Input: part model. Units: mm. Frame: model coordinates. Face numbers are marked on the shaded views. Coordinates: 2 decimals unless noted, no trailing zeros. Loops run counter-clockwise (first coordinate to the right, second up) from the corner with the lowest first, then second, coordinate; pieces in that order, holes last. Notation, with made-up numbers: (13.25, 27.25) -> (35.25, 27.25) arc R18 ccw to (35.25, 55.25) -> close; hole circle Ø3 at (78, 41). An arc over 180 degrees is marked (long way). Answer as a JSON object with one key per item and string values.
Autodesk Inventor part; units mm, degrees
ref_plane "YZ Plane" through (0, 0, 0) normal (1, 0, 0) x (0, 1, 0)
ref_plane "XZ Plane" through (0, 0, 0) normal (0, 1, 0) x (-1, 0, 0)
ref_plane "XY Plane" through (0, 0, 0) normal (0, 0, 1) x (1, 0, 0)
sketch "Эскиз1" plane through (0, 0, 0) normal (0, 1, 0) x (-1, 0, 0)
  circle A0 centre (0, 0) radius 2.5
  circle A1 centre (0, 0) radius 7.5
  line L0 (0, 7.5) -> (7.5, 7.5)
  line L1 (7.5, 7.5) -> (7.5, -7.5)
  line L2 (7.5, -7.5) -> (0, -7.5)
  line L3 (0, -7.5) -> (0, 7.5)
  line L4 (-7.5, 0) -> (-12.5, 0)
  circle A2 centre (-12.5, 0) radius 2.6
  circle A3 centre (-12.5, 0) radius 5
  line L5 (-1.5661, 7.3347) -> (-13.4999, 4.899)
  line L6 (-13.5, -4.899) -> (-1.5, -7.3485)
  dimension "d0" = 5
  dimension "d1" = 15
  dimension "d2" = 5
  dimension "d3" = 5.2
extrude "Выдавливание1" add sketch "Эскиз1" along normal blind 2 contours A0 L3 A1 | A0 L3 A1 | L0 L1 A1 | A1 L1 L2 | A1 A3 L5 | L6 A3 A1 | A3
fillet "Сопряжение1" radius 0.7 8 edges at (0.7874, 0, 7.4586) (-3.75, 0, 7.5) (-7.5, 0, 0) (0.7538, 0, -7.462) (7.5, 0, -6.1237) (17.5, 0, 0.0001) (7.533, 0, 6.1168) (-3.75, 0, -7.5)
properties part number "block_02"
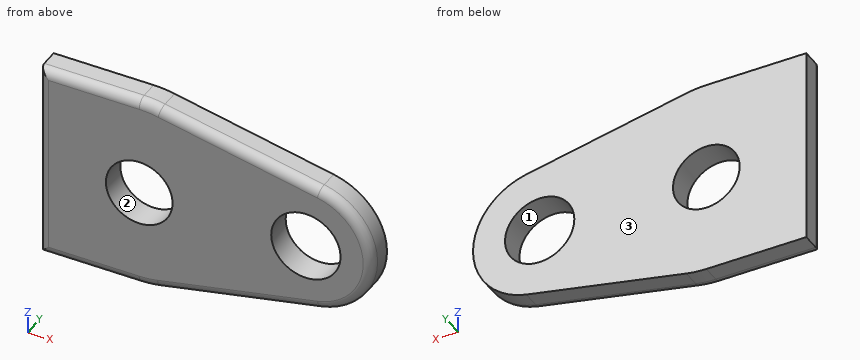
1. Pin query (flat end, axial travel): P1, Ø5, axis at x = 6.5, z = -3.5, coming from the -Y side; P2, Ø4.5, axis at x = 0, z = 0, coming from the +Y side; P3, Ø1, axis at x = 2.5, y = 0.5, coming from the +Z side. Return the tip coordinate at first contact, or that it passes through.
Reply:
{"P1": "stops at y = 0", "P2": "passes through", "P3": "stops at z = 7.24"}
2. Section query A-A (y = 1.3). Return loops of the section in (x, z).
Reply:
{"outline": "(-7.5, -7.5) -> (0, -7.5) arc R7.5 ccw to (1.5, -7.35) -> (13.5, -4.9) arc R5 ccw to (13.5, 4.9) -> (1.57, 7.33) arc R7.5 ccw to (0, 7.5) -> (-7.5, 7.5) -> close; hole circle Ø5 at (0, 0); hole circle Ø5.2 at (12.5, 0)"}
3. Line query: line 1 along X through (y, z) = (1.65, -1.75); line 2 along X through (y, z) = (0.6, -1); line 3 along Z through (x, y) = (0, 1.1). Output: solid intervals per line, ascending.
Reply:
{"line 1": "x = -7.5 to -1.79, 1.79 to 10.58, 14.42 to 17.18", "line 2": "x = -7.49 to -2.29, 2.29 to 10.1, 14.9 to 17.39", "line 3": "z = -7.5 to -2.5, 2.5 to 7.5"}
4. Mould query, pull axis X, two halves, no side actions, for the marked faces 1, 2 and 3. Classes: pulls with the +X half, pulls with the -X half, needs draft (parallel to the pull), parting line crosses it, or undercut.
Reply:
{"face 1": "undercut", "face 2": "undercut", "face 3": "needs draft"}
5. Section query B-B (z = 0). Return loops of the section in (x, y), plus the area to 3 significant figures.
Reply:
{"outline": "(-7.5, 0.7) arc R0.7 ccw to (-6.8, 0) -> (-2.5, 0) -> (-2.5, 2) -> (-7.5, 2) -> close; (2.5, 0) -> (9.9, 0) -> (9.9, 2) -> (2.5, 2) -> close; (15.1, 0) -> (16.8, 0) arc R0.7 ccw to (17.5, 0.7) -> (17.5, 2) -> (15.1, 2) -> close", "area": "29.4 mm2"}
